Part model, mm, in its own coordinate system. Face numbers are marked on the shaded views. A direction names the side the tool comes from. Round coordinates to 2 decimals unless told otherwise and drop trailing zeros. Loops run counter-clockwise (first coordinate to the right, second up) from the corner with the lowest first, then second, coordinate; pieces in that order, holes last. Notation, with made-up numbers: M 56,51 L 101,51 A26 ccw 101,66 Z; hole C 42,1.5 d9. An arc over 180 degrees is marked long. Write each question's results on one line, items separated by ' | '.
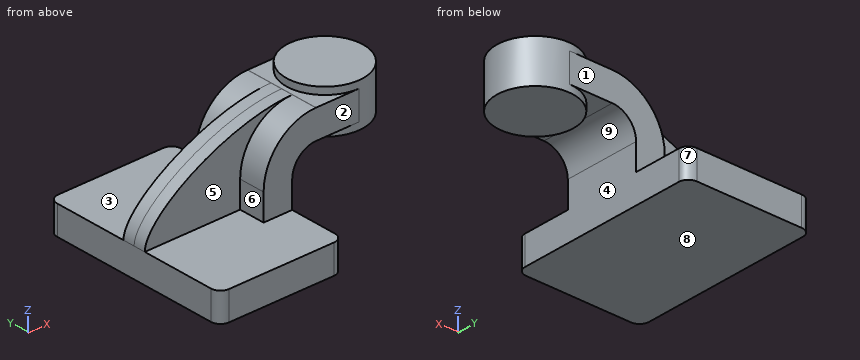
from build123d import *

# Parameters (mm, degrees)
F1_DEPTH = 63.5
F0_W     = 25.4
F0_H     = 19.05
F2_DEPTH = 25.4
F3_DEPTH = 7.9375
F5_R     = 6.35


with BuildPart() as f1:
    # F0 (on Front) → F1 (new body, symmetric)
    with BuildSketch(Plane.XZ):
        Polygon((-41.275, 9.525), (-41.275, -9.525), (41.275, -9.525), (41.275, 9.525), (22.225, 9.525), align=None)
    extrude(amount=F1_DEPTH, both=True)

    # F0 (on Front) → F2 (join, symmetric)
    with BuildSketch(Plane.XZ):
        with BuildLine():
            Line((22.225, 9.525), (41.275, 9.525))
            Line((41.275, 9.525), (41.275, 27.0002))
            ThreePointArc((41.275, 27.0002), (45.9246798487, 38.2255201513), (57.15, 42.8752))
            Line((57.15, 42.8752), (60.325, 42.8752))
            Line((60.325, 42.8752), (60.325, 61.9252))
            Line((60.325, 61.9252), (57.15, 61.9252))
            ThreePointArc((57.15, 61.9252), (57.0327801624, 61.9250032852), (56.9155616453, 61.924413143))
            ThreePointArc((56.9155616453, 61.924413143), (32.3715478234, 51.6128782925), (22.225, 27.0002))
            Line((22.225, 27.0002), (22.225, 9.525))
        make_face()
        with Locations((73.025, 52.4002)):
            Rectangle(F0_W, F0_H)
    extrude(amount=F2_DEPTH, both=True)

    # F0 (on Front) → F3 (join, symmetric)
    with BuildSketch(Plane.XZ):
        with BuildLine():
            add(Edge.make_bspline(
                [(-41.275, 9.525), (-40.772556892, 29.51723469), (13.8574212283, 61.721808406), (56.9155616453, 61.924413143)],
                knots=[0, 0, 0, 0, 111.3024346727, 111.3024346727, 111.3024346727, 111.3024346727], degree=3))
            Line((-41.275, 9.525), (22.225, 9.525))
            Line((22.225, 9.525), (22.225, 27.0002))
            ThreePointArc((22.225, 27.0002), (32.3715478234, 51.6128782925), (56.9155616453, 61.924413143))
        make_face()
    extrude(amount=F3_DEPTH, both=True)

    # F0 (on Front) → F4 (revolve)
    with BuildSketch(Plane.XZ):
        Polygon((85.725, 66.675), (85.725, 61.9252), (85.725, 42.8752), (85.725, 38.1), (111.125, 38.1), (111.125, 66.675), align=None)
    revolve(axis=Axis((85.725, 0, 52.3875), (0, 0, 1)))

    # F5
    f5_edges = [f1.edges().sort_by_distance(p)[0] for p in [
        (41.275, -63.5, 0),
        (41.275, 63.5, 0),
        (-41.275, -63.5, 0),
        (-41.275, 63.5, 0),
    ]]
    fillet(f5_edges, radius=F5_R)


solid = f1.part
Item 1: Band-saw the part on C-C on x = 71. Give the cut face in (y, z) (3 decimals).
Filled sheet:
outline: M -25.4,42.875 L -20.696,42.875 L -20.696,38.1 L 20.696,38.1 L 20.696,42.875 L 25.4,42.875 L 25.4,61.925 L 20.696,61.925 L 20.696,66.675 L -20.696,66.675 L -20.696,61.925 L -25.4,61.925 Z
Item 2: Which spindle directions (+Z, -Z, +X, -X, +Y, -Y) get a long thin tool onto all of the face, cutting with end or side? Do the marked faces 1, 2, 3, 4 and 5. Say none if no direction does.
Filled sheet:
face 1: +Z, +X, -X, +Y | face 2: +Z, +X, -X, -Y | face 3: +Z, -X, +Y | face 4: -Z, +X, +Y, -Y | face 5: +Z, -X, -Y
Item 3: Band-saw the part on A-A on z = 7. Give the cut face in (x, y) (3 decimals).
Filled sheet:
outline: M -41.275,-57.15 A6.35 ccw -34.925,-63.5 L 34.925,-63.5 A6.35 ccw 41.275,-57.15 L 41.275,57.15 A6.35 ccw 34.925,63.5 L -34.925,63.5 A6.35 ccw -41.275,57.15 Z
Item 4: Band-saw the part on D-D on y = -12. Give the cut face in (x, z) (3 decimals).
Filled sheet:
outline: M -41.275,-9.525 L 41.275,-9.525 L 41.275,27 A15.875 cw 57.15,42.875 L 63.338,42.875 L 63.338,38.1 L 108.112,38.1 L 108.112,66.675 L 63.338,66.675 L 63.338,61.925 L 57.15,61.925 A34.925 ccw 22.225,27 L 22.225,9.525 L -41.275,9.525 Z
Item 5: Two-plate mould, pull along X, no slides. Class the marked faces 6, 7, 8 and 9: +X half, -X half, draft (parallel to the pull), parting line (faces both ways), or undercut.
Filled sheet:
face 6: -X half | face 7: +X half | face 8: draft | face 9: undercut
Item 6: Band-saw the part on B-B on y = 30.5. Give the cut face in (x, z) (3 decimals).
Filled sheet:
outline: M -41.275,-9.525 L 41.275,-9.525 L 41.275,9.525 L -41.275,9.525 Z
Item 7: Drop flat-ended pins along their axis: P1, Ø10, axis at x = 68.5, z = 48, coming from the -Y side; P2, Ø15.5, axis at x = -14, z = 33, coming from the +Y side; P3, Ø14, axis at y = 20, z = 18, coming from the -X side (3 decimals). Give the stop position or say it passes through.
Filled sheet:
P1: y = -25.4 | P2: y = 7.94 | P3: x = 22.225
Item 8: Wall check: L1, parallel to Y at x = 77.5, z = 43; L2, parallel to Y at x = 5.5, z = 39.5; L3, parallel to Z at x = 12, y = -37.5 (3 decimals). Give the ranges that are in metal, low to high.
Filled sheet:
L1: -25.4 to 25.4 | L2: -7.94 to 7.94 | L3: -9.525 to 9.525
